Verification items for the finished model (mm, model axes). Round coordinates to 2 decimals unless told otherwise and drop trailing zeros. One line per item, written item: value.
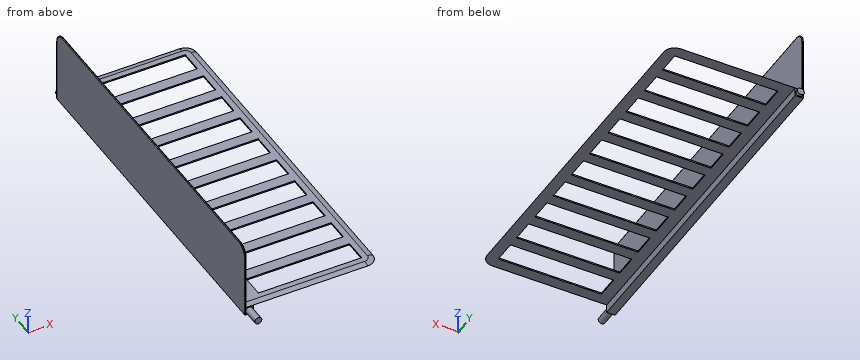
from build123d import *

# Parameters (mm, degrees)
F0_W         = 6.35
F0_H         = 298.45
F0_W_2       = 603.25
F0_H_2       = 6.35
F1_DEPTH     = 1574.8
F2_W         = 38.1
F2_H         = 38.1
F3_DEPTH     = 1574.8
F4_R         = 15.875
F5_DEPTH     = 76.2
F6_R         = 15.875
F7_DEPTH     = 12.7
F8_W         = 469.9
F8_H         = 101.6
F9_DEPTH     = 25.4
F10_R        = 50.8
F11_T1_DEPTH = 1473.2
F11_T3_DEPTH = 552.45
F11_T6_ANGLE = 90
F11_T8_ANGLE = 90
F12_R        = 3.17499


# Not quite as in the source:
# - a fillet or chamfer that OpenCascade refuses, or shapes differently, is made with other operations: its cross-section is extruded or revolved along the edge and cut away or added
# - a fillet or chamfer is up to 0.001 mm smaller than in the source, because OpenCascade refuses the exact size


with BuildPart() as f1:
    # F0 (on Front) → F1 (new body)
    with BuildSketch(Plane.XZ):
        with Locations((3.175, 155.575)):
            Rectangle(F0_W, F0_H)
        with Locations((307.975, 3.175)):
            Rectangle(F0_W_2, F0_H_2)
        with Locations((3.175, 3.175)):
            Rectangle(F0_W, F0_H_2)
    extrude(amount=F1_DEPTH)

    # F2 (on face) → F3 (join)
    with BuildSketch(Plane.XZ.offset(1574.8)):
        with Locations((19.05, -19.05)):
            Rectangle(F2_W, F2_H)
    extrude(amount=-F3_DEPTH)

    # F4 (on face) → F5 (join)
    with BuildSketch(Plane.XZ.offset(1574.8)):
        with Locations((19.05, -19.05)):
            Circle(F4_R)
    extrude(amount=F5_DEPTH)

    # F6 (on face) → F7 (join)
    with BuildSketch(Plane(origin=(0, 0, 0), x_dir=(-1, 0, 0), z_dir=(0, 1, 0))):
        with Locations((-19.05, -19.05)):
            Circle(F6_R)
    extrude(amount=F7_DEPTH)

    # F8 (on face) → F9 (cut)
    with BuildSketch(Plane(origin=(0, 0, 0), x_dir=(1, 0, 0), z_dir=(0, 0, -1))):
        with Locations((323.85, 1473.2)):
            Rectangle(F8_W, F8_H)
        with Locations((323.85, 1320.8)):
            Rectangle(F8_W, F8_H)
        with Locations((323.85, 1168.4)):
            Rectangle(F8_W, F8_H)
        with Locations((323.85, 1016)):
            Rectangle(F8_W, F8_H)
        with Locations((323.85, 863.6)):
            Rectangle(F8_W, F8_H)
        with Locations((323.85, 711.2)):
            Rectangle(F8_W, F8_H)
        with Locations((323.85, 558.8)):
            Rectangle(F8_W, F8_H)
        with Locations((323.85, 406.4)):
            Rectangle(F8_W, F8_H)
        with Locations((323.85, 254)):
            Rectangle(F8_W, F8_H)
        with Locations((323.85, 101.6)):
            Rectangle(F8_W, F8_H)
    extrude(amount=-F9_DEPTH, mode=Mode.SUBTRACT)

    # F10
    f10_edges = [f1.edges().sort_by_distance(p)[0] for p in [
        (609.6, 0, 3.175),
        (609.6, -1574.8, 3.175),
        (3.175, -1574.8, 304.8),
        (3.175, 0, 304.8),
    ]]
    fillet(f10_edges, radius=F10_R)

    # F11: fillet of radius 50.8 on 1 edges, made by hand

    # F11_s2 → F11_t1 (cut)
    with BuildSketch(Plane.XZ.offset(50.8)):
        with BuildLine():
            ThreePointArc((585.0065557516, 6.35), (597.7065557516, 4.7368884968), (609.6, 0))
            Line((609.6, 0), (609.6, 6.35))
            Line((609.6, 6.35), (585.0065557516, 6.35))
        make_face()
    extrude(amount=F11_T1_DEPTH, mode=Mode.SUBTRACT)

    # F11_s4 → F11_t3 (cut)
    with BuildSketch(Plane.YZ.offset(6.35)):
        with BuildLine():
            ThreePointArc((-1574.8, 0), (-1562.9065557516, 4.7368884968), (-1550.2065557516, 6.35))
            Line((-1550.2065557516, 6.35), (-1574.8, 6.35))
            Line((-1574.8, 6.35), (-1574.8, 0))
        make_face()
        with BuildLine():
            ThreePointArc((0, 0), (-11.8934442484, 4.7368884968), (-24.5934442484, 6.35))
            Line((-24.5934442484, 6.35), (0, 6.35))
            Line((0, 6.35), (0, 0))
        make_face()
    extrude(amount=F11_T3_DEPTH, mode=Mode.SUBTRACT)

    # F11_s5 → F11_t6 (revolve, cut)
    with BuildSketch(Plane.YZ.offset(558.8)):
        with BuildLine():
            ThreePointArc((-24.5934442484, 6.35), (-11.8934442484, 4.7368884968), (0, 0))
            Line((0, 0), (0, 6.35))
            Line((0, 6.35), (-24.5934442484, 6.35))
        make_face()
    revolve(axis=Axis((558.8, -50.8, 6.35), (0, 0, -1)), revolution_arc=F11_T6_ANGLE, mode=Mode.SUBTRACT)

    # F11_s7 → F11_t8 (revolve, cut)
    with BuildSketch(Plane.YZ.offset(558.8)):
        with BuildLine():
            ThreePointArc((-1550.2065557516, 6.35), (-1562.9065557516, 4.7368884968), (-1574.8, 0))
            Line((-1574.8, 0), (-1574.8, 6.35))
            Line((-1574.8, 6.35), (-1550.2065557516, 6.35))
        make_face()
    revolve(axis=Axis((558.8, -1524, 6.35), (0, 0, 1)), revolution_arc=F11_T8_ANGLE, mode=Mode.SUBTRACT)

    # F12 (radius 3.175 in the source; OpenCascade refuses exactly that, so slightly less here)
    f12_edges = [f1.edges().sort_by_distance(p)[0] for p in [
        (6.35, -787.4, 304.8),
        (0, -787.4, 304.8),
        (0, -14.878976, 289.921024),
        (0, -1559.921024, 289.921024),
        (0, 0, 107.95),
        (0, -1574.8, 107.95),
        (6.35, -14.878976, 289.921024),
        (6.35, -1559.921024, 289.921024),
        (6.35, 0, 127),
        (6.35, -1574.8, 127),
    ]]
    fillet(f12_edges, radius=F12_R)


solid = f1.part
(1) Thickness scan on L1, parallel to X at y = -671, z = 204; L2, parallel to Z at x = 25.5, y = -403. Record the ranges inside material, lowest first. Write a range as from..to.
Completed:
L1: x = 0..6.35
L2: z = -38.1..6.35
(2) Sectioned sample at C-C on x = 379.5. Count the separate pieces of the cut face and the enclosed holes in it, and give its area (3 significant figures).
Completed:
separate pieces: 11
enclosed holes: 0
area: 3,450 mm^2
(3) Depth check by flat-ended pin: pin 1 Ø1.9 at (x, z) = (303, 3) entering from -Y; pin 2 Ø5 at (y, z) = (-862.5, 82.5) entering from +X; pin 3 Ø1.9 at (y, z) = (-111, 2.5) entering from +X. Enter the tip coordinate at first touch or a pass-through.
Completed:
pin 1: stops at y = -1570.66
pin 2: stops at x = 6.35
pin 3: stops at x = 606.56
